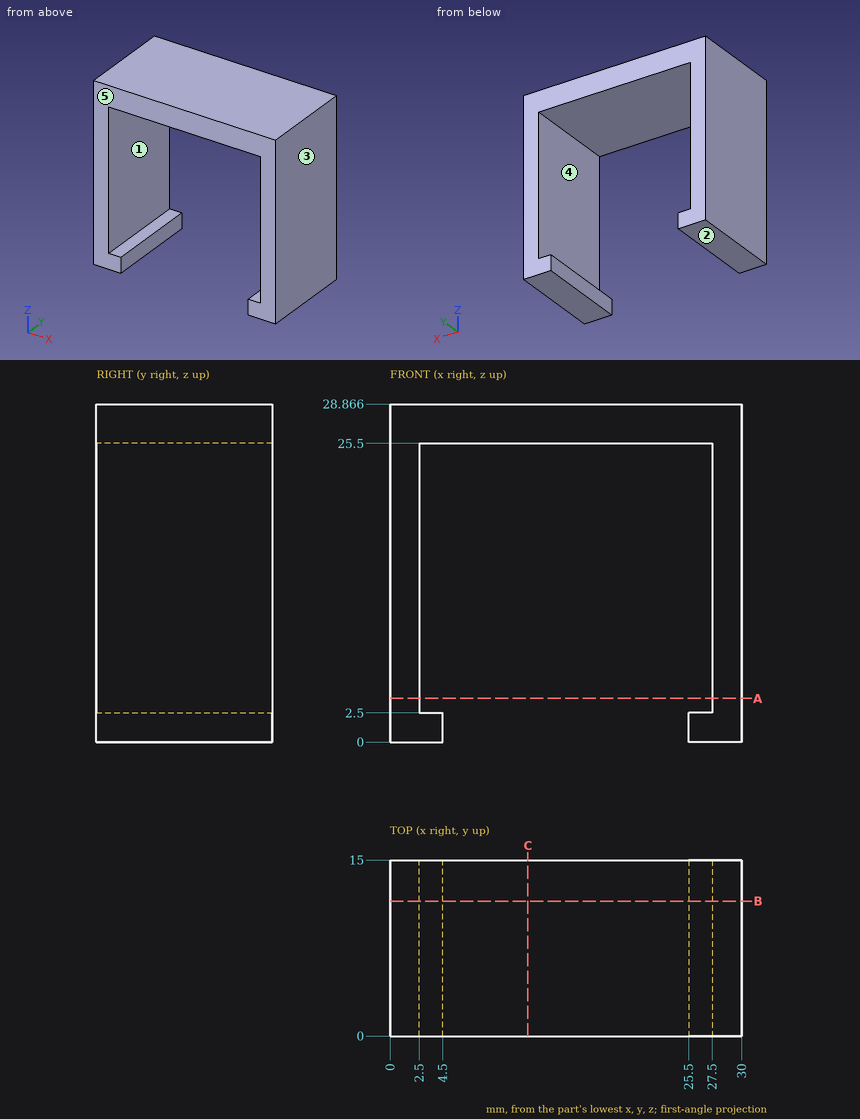
Design review of the part shown in the three views and the two pictorial views. Dimensions are in mm from the part's minimum x, y and z. A direction names the side the tool comes from. Round coordinates to 2 decimals unless told otherwise and drop trailing zeros. Order: outer loops, then holes, each group sorted by start corner. A loop starts at its lowest first (then second) coordinate and runs counter-clockwise, first axis right, second up. Notation, with made-up numbers: (-20, 60.5) - (17, 60.5) arc R23 cw to (17, 79.5) - close; hole circle Ø4 at (-29.75, 34). An arc over 180 degrees is marked (long way). Answer in a Markdown table with one row per item.
(1) Machinability: for the marked faces 1 and 2, which of the approach directions +Z, -Z, +X, -X, +Y, -Y give a long, thin tool a straight path to every point of the face, cutting with its end or side? Answer none if there is none.
Result set:
| item | result |
|---|---|
| face 1 | +Y, -Y |
| face 2 | -Z, +X, -X, +Y, -Y |
(2) Take a section at B-B on y = 11.5. Write out the cut boundary in (x, z).
Result set:
| item | result |
|---|---|
| outline | (0, 0) - (4.5, 0) - (4.5, 2.5) - (2.5, 2.5) - (2.5, 25.5) - (27.5, 25.5) - (27.5, 2.5) - (25.5, 2.5) - (25.5, 0) - (30, 0) - (30, 28.87) - (0, 28.87) - close |
(3) Clearance check with a flat-ended pin moving along its axis: P1, Ø3, axis at x = 19, y = 5, coming from the -Z side. State where the tip first meets the part, or that it passes through.
Result set:
| item | result |
|---|---|
| P1 | stops at z = 25.5 |
(4) For line 1 (X direction, y = 8.25, z = 24); line 2 (Z direction, x = 8.5, y = 8.75), list the stretches that pass through material, from the lowest coordinate up. Write a range as from..to.
Result set:
| item | result |
|---|---|
| line 1 | x = 0..2.5, 27.5..30 |
| line 2 | z = 25.5..28.87 |
(5) Take a section at A-A on z = 3.75. Write out the cut boundary in (x, y).
Result set:
| item | result |
|---|---|
| outline | (0, 0) - (2.5, 0) - (2.5, 15) - (0, 15) - close; (27.5, 0) - (30, 0) - (30, 15) - (27.5, 15) - close |
(6) Take a section at C-C on x = 11.75. Write out the cut boundary in (y, z), plus the area to 3 significant figures.
Result set:
| item | result |
|---|---|
| outline | (0, 25.5) - (15, 25.5) - (15, 28.87) - (0, 28.87) - close |
| area | 50.5 mm2 |
(7) Mouldability with a two-part tool opening along X and no side actions: class the marked faces 3, 4 and 5 as released by +X, released by -X, zero draft, split by the parting line, or undercut.
Result set:
| item | result |
|---|---|
| face 3 | released by +X |
| face 4 | undercut |
| face 5 | zero draft |
